from build123d import *

# Parameters (mm, degrees)
F0_R          = 18
F0_R_2        = 16.5
F1_DEPTH      = 25
F2_R          = 7.5
F3_DEPTH      = 488
F4_END_RADIUS = 16.5
F3_FACE_R     = 7.5
F4_REACH      = 509.2142035356


with BuildPart() as f1:
    # F0 (on Front) → F1 (new body)
    with BuildSketch(Plane.XZ):
        Circle(F0_R)
        Circle(F0_R_2, mode=Mode.SUBTRACT)
    extrude(amount=F1_DEPTH)

    # F2 (on Top) → F3 (join)
    with BuildSketch(Plane.XY):
        with Locations((0, -12.5)):
            Circle(F2_R)
    extrude(amount=F3_DEPTH)

    f4_end = (Plane.ZX.offset(-12.5) * Cylinder(F4_END_RADIUS, 2034.2177557588, mode=Mode.PRIVATE)).faces().sort_by_distance((-16.5, -12.5, 0))[0]
    # F3_face (on face) → F4 (cut, up to the whole of a round face its end follows)
    with BuildSketch(Plane(origin=(0, -12.5, 0), x_dir=(1, 0, 0), z_dir=(0, 0, -1))):
        Circle(F3_FACE_R)
    f4_long = extrude(amount=-F4_REACH, mode=Mode.PRIVATE)
    add(split(f4_long, bisect_by=f4_end, keep=Keep.BOTTOM, mode=Mode.PRIVATE), mode=Mode.SUBTRACT)


solid = f1.part
Source: CAD feature listing. Evaluate the final solid. Frame: model axes, mm. A direction names the side the tool comes from. Round coordinates to 2 decimals unless told otherwise and drop trailing zeros. Order: outer loops, then holes, each group sorted by start corner. A loop starts at its lowest first (then second) coordinate and runs counter-clockwise, first axis right, second up. Notation, with made-up numbers: (79, 38) - (130, 38) arc R29 ccw to (130, 63) - close; hole circle Ø1 at (29, 86.5). An arc over 180 degrees is marked (long way). Use a Markdown table: item, result. Add a question column.
1. Section query A-A (x = 0). Return the cut outline in (y, z).
2. Section query D-D (z = 398). Return the cut outline in (x, y), then the cut area to 3 significant figures.
3. First-contact query: pin 1 (12 mm diameter, centred on x = 13, y = -7.5, fed in from -Z); pin 2 (12 mm diameter, centred on y = -15, z = 344, fed in from -X); pin 3 (1.5 mm diameter, centred on x = 1, z = 398, fed in from +Y). Flat tips, straight axial feed; report the tip coordinate or a pass-through.
4. Section query C-C (y = -12.5). Return the cut outline in (x, z).
5. Mould query, pull axis X, two halves, no side actions, for faces 3 (the flat face through (8, -25, -15)), 4 (the cylindrical face through (-3.902, -12.325, -17.572)), 5 (the cylindrical face through (15.24, -12.32, -6.32)). Classes: +X half, -X half, draft (parallel to the pull), parting line (faces both ways), or undercut.
6. Set-up query: faces 1 (the cylindrical face through (-1.63, -19.82, 248.88)), 2 (the flat face through (0, -12, 488)). Return all of +Z, -Z, +X, -X, +Y, -Y with unobstructed straight access to the full face (end or side cutting, diameter ignored); none if empty.
7. Line query: probe 1 along Z at (x, y) = (0, -19); probe 2 along X at (y, z) = (-12.5, 383); probe 3 along Z at (x, y) = (-9.5, -22.75). Output: solid intervals per line, ascending.
8. Section query B-B (z = 0). Return the cut outline in (x, y), then the cut area to 3 significant figures.
Derived:
| question | item | result |
|---|---|---|
| 1 | outline | (-25, -18) - (0, -18) - (0, -16.5) - (-25, -16.5) - close; (-25, 16.5) - (0, 16.5) - (0, 18) - (-5, 18) - (-5, 488) - (-20, 488) - (-20, 18) - (-25, 18) - close |
| 2 | outline | circle Ø15 at (0, -12.5) |
| 2 | area | 177 mm2 |
| 3 | pin 1 | z = -16.58 |
| 3 | pin 2 | x = -7.5 |
| 3 | pin 3 | y = -5 |
| 4 | outline | (-7.5, 16.36) arc R18 ccw (long way) to (7.5, 16.36) - (7.5, 488) - (-7.5, 488) - close; hole circle Ø33 at (0, 0) |
| 5 | face 3 | draft |
| 5 | face 4 | parting line |
| 5 | face 5 | undercut |
| 6 | face 1 | +Z |
| 6 | face 2 | +Z, +X, -X, +Y, -Y |
| 7 | probe 1 | -18 to -16.5, 16.5 to 488 |
| 7 | probe 2 | -7.5 to 7.5 |
| 7 | probe 3 | -15.29 to -13.49, 13.49 to 15.29 |
| 8 | outline | (-18, -25) - (-16.5, -25) - (-16.5, 0) - (-18, 0) - close; (16.5, -25) - (18, -25) - (18, 0) - (16.5, 0) - close |
| 8 | area | 75.0 mm2 |
